Could you check a few things on this model? Use its own coordinates, in mm. Round coordinates to 2 decimals unless told otherwise and drop trailing zeros. Write each loop counter-clockwise with the first axis right and the second up, starting at its lowest first coordinate (ties: lowest second). Pieces come first, ordered by that corner, then holes. Notation, with made-up numbers: M 28.25,80 L 68.25,80 A18 ccw 68.25,96 Z; hole C -40,22.25 d5. An arc over 180 degrees is marked long. One line per item, written item: value. Start each with the question number.
(1) Thinking about a two-plate mould opening in Y: for faces 1 (the face through (-8.071, -61.472, 1.479)), 2 (the face through (-15, -13, 3)), 3 (the face through (-12.75, 26.74, 1.52)), which applies, released by +Y, released by -Y, zero draft, split by the parting line, or undercut?
(2) I want a section at B-B on x = 23.5. Please give me the cut outline in (y, z), and give its area (3 significant figures).
(3) I want a section at A-A on x = -6.5. Please give me the cut outline in (y, z), and give its area (3 significant figures).
(4) If I drill on L1, parallel to Y at x = 23.5, z = 0.85; L2, parallel to Y at x = -25, z = 2.2; L3, parallel to X at y = -22, z = 1.6, over which ranges is the centre line in solid material (lowest first)?
(5) I'm going to push flat-ended pins straight in: pin 1 Ø2.5 at (x, y) = (23.5, -23.5) entering from +Z; pin 2 Ø1.5 at (y, z) = (-28, 2) entering from +X. Where does each tip first touch, or does it pass through?
(6) I want a section at D-D on y = 55. Please give me the cut outline in (x, z), and give its area (3 significant figures).
Autodesk Inventor part; units mm, degrees
ref_plane "YZ Plane" through (0, 0, 0) normal (1, 0, 0) x (0, 1, 0)
ref_plane "XZ Plane" through (0, 0, 0) normal (0, 1, 0) x (-1, 0, 0)
ref_plane "XY Plane" through (0, 0, 0) normal (0, 0, 1) x (1, 0, 0)
sketch "Sketch1" plane through (0, 0, 0) normal (0, 0, 1) x (1, 0, 0)
  circle A0 centre (0, 55) radius 2.65
  arc A1 (62, 0) -> (-62, 0) centre (0, 0) ccw
  line L0 (-62, 0) -> (-62, -80)
  line L1 (-62, -80) -> (62, -80)
  line L2 (62, -80) -> (62, 0)
  circle A2 centre (0, 0) radius 47.5 construction
  circle A3 centre (0, 0) radius 55 construction
  line L3 (0, 55) -> (0, 0) construction
  circle A4 centre (-52.308108, 16.995935) radius 2.65
  circle A5 centre (-32.328189, -44.495935) radius 2.65
  circle A6 centre (32.328189, -44.495935) radius 2.65
  circle A7 centre (52.308108, 16.995935) radius 2.65
  dimension "d23" = 110
  dimension "d24" = 95
  dimension "d25" = 62
  dimension "d26" = 80
  dimension "d27" = 5.3
  dimension "d30" = 360
extrude "Extrusion1" add sketch "Sketch1" along normal blind 3
sketch "Sketch2" plane through (0, 0, 3) normal (0, 0, 1) x (1, 0, 0)
  circle A0 centre (0, 0) radius 19.5
  line L0 (-23.5, -23.5) -> (23.5, -23.5) construction
  line L1 (23.5, -23.5) -> (23.5, 23.5) construction
  line L2 (23.5, 23.5) -> (-23.5, 23.5) construction
  line L3 (-23.5, 23.5) -> (-23.5, -23.5) construction
  line L4 (-23.5, -23.5) -> (23.5, 23.5) construction
  line L5 (23.5, -23.5) -> (-23.5, 23.5) construction
  circle A1 centre (-23.5, 23.5) radius 2
  circle A2 centre (23.5, 23.5) radius 2
  circle A3 centre (23.5, -23.5) radius 2
  circle A4 centre (-23.5, -23.5) radius 2
  dimension "d2" = 39
  dimension "d3" = 47
  dimension "d4" = 4
extrude "Extrusion2" cut sketch "Sketch2" against normal through all
sketch "Sketch3" plane through (0, 0, 3) normal (0, 0, 1) x (1, 0, 0)
  arc A0 (62, 0) -> (-62, 0) centre (0, 0) ccw
  circle A1 centre (0, 0) radius 62
  circle A2 centre (0, 0) radius 147.62847
  point P0 (62, 0)
sketch "Sketch3 outline for Extrusion3" plane through (0, 0, 3) normal (0, 0, 1) x (1, 0, 0)
  circle A0 centre (0, 0) radius 147.62847
  arc A1 (62, 0) -> (-62, 0) centre (0, 0) cw
  arc A2 (-62, 0) -> (62, 0) centre (0, 0) cw
extrude "Extrusion3" cut sketch "Sketch3 outline for Extrusion3" against normal through all
sketch "Sketch4" plane through (0, 0, 3) normal (0, 0, 1) x (1, 0, 0)
  circle A0 centre (0, 0) radius 30 construction
  circle A1 centre (-27.716386, 11.480503) radius 1.6
  line L0 (-27.716386, 11.480503) -> (0, 0) construction
  line L1 (-27.716386, -11.480503) -> (0, 0) construction
  circle A2 centre (-27.716386, -11.480503) radius 1.6
  line L2 (-11.480503, -27.716386) -> (0, 0) construction
  circle A3 centre (-11.480503, -27.716386) radius 1.6
  line L3 (11.480503, -27.716386) -> (0, 0) construction
  circle A4 centre (11.480503, -27.716386) radius 1.6
  line L4 (27.716386, -11.480503) -> (0, 0) construction
  circle A5 centre (27.716386, -11.480503) radius 1.6
  line L5 (27.716386, 11.480503) -> (0, 0) construction
  circle A6 centre (27.716386, 11.480503) radius 1.6
  line L6 (11.480503, 27.716386) -> (0, 0) construction
  circle A7 centre (11.480503, 27.716386) radius 1.6
  line L7 (-11.480503, 27.716386) -> (0, 0) construction
  circle A8 centre (-11.480503, 27.716386) radius 1.6
  line L8 (0, 0) -> (-27.716386, 0) construction
  line L9 (-27.716386, 0) -> (-27.716386, 11.480503) construction
  line L10 (-27.716386, 0) -> (-27.716386, -11.480503) construction
  dimension "d9" = 60
  dimension "d10" = 3.2
  dimension "d13" = 360
extrude "Extrusion4" cut sketch "Sketch4" against normal through all
properties part number "J0_motorbracket"
Found:
1. face 1: split by the parting line
1. face 2: zero draft
1. face 3: undercut
2. outline: M -57.37,0 L -25.5,0 L -25.5,3 L -57.37,3 Z; M -21.5,0 L 21.5,0 L 21.5,3 L -21.5,3 Z; M 25.5,0 L 57.37,0 L 57.37,3 L 25.5,3 Z
2. area: 320 mm²
3. outline: M -61.66,0 L -18.38,0 L -18.38,3 L -61.66,3 Z; M 18.38,0 L 61.66,0 L 61.66,3 L 18.38,3 Z
3. area: 260 mm²
4. L1: y = -57.37 to -25.5, -21.5 to 21.5, 25.5 to 57.37
4. L2: y = -56.74 to -24.82, -22.18 to 22.18, 24.82 to 56.74
4. L3: x = -57.97 to -24.82, -22.18 to 22.18, 24.82 to 57.97
5. pin 1: passes through
5. pin 2: stops at x = 55.69
6. outline: M -28.62,0 L -2.65,0 L -2.65,3 L -28.62,3 Z; M 2.65,0 L 28.62,0 L 28.62,3 L 2.65,3 Z
6. area: 156 mm²
